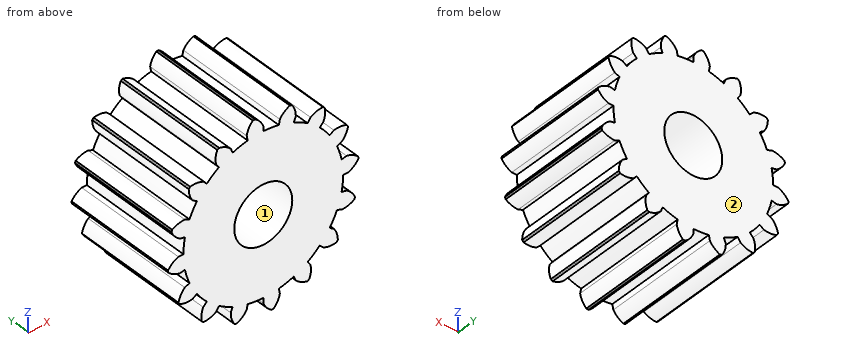
from build123d import *

# Parameters (mm, degrees)
F0_R     = 1.5875
F1_DEPTH = 6.35


with BuildPart() as f1:
    # F0 (on Front) → F1 (new body)
    with BuildSketch(Plane.XZ):
        with BuildLine():
            ThreePointArc((0, 4.653198), (-0.181622, 4.967595), (-0.451324, 5.210686))
            ThreePointArc((-0.451324, 5.210686), (-0.481995, 5.207938), (-0.512649, 5.20501))
            ThreePointArc((-0.512649, 5.20501), (-0.543285, 5.201901), (-0.573903, 5.198613))
            ThreePointArc((-0.573903, 5.198613), (-0.790998, 4.907577), (-0.907794, 4.563788))
            Line((-0.907794, 4.563788), (-0.853047, 4.288558))
            ThreePointArc((-0.853047, 4.288558), (-1.269292, 4.184294), (-1.673312, 4.039734))
            Line((-1.673312, 4.039734), (-1.780702, 4.298995))
            ThreePointArc((-1.780702, 4.298995), (-2.068813, 4.519956), (-2.411012, 4.641332))
            ThreePointArc((-2.411012, 4.641332), (-2.438297, 4.627056), (-2.465497, 4.61262))
            ThreePointArc((-2.465497, 4.61262), (-2.492612, 4.598024), (-2.51964, 4.583269))
            ThreePointArc((-2.51964, 4.583269), (-2.608835, 4.231308), (-2.585178, 3.868993))
            Line((-2.585178, 3.868993), (-2.429273, 3.635664))
            ThreePointArc((-2.429273, 3.635664), (-2.773933, 3.380047), (-3.091878, 3.091878))
            Line((-3.091878, 3.091878), (-3.290308, 3.290308))
            ThreePointArc((-3.290308, 3.290308), (-3.641046, 3.384194), (-4.003645, 3.365377))
            ThreePointArc((-4.003645, 3.365377), (-4.02339, 3.341747), (-4.042995, 3.318))
            ThreePointArc((-4.042995, 3.318), (-4.06246, 3.294139), (-4.081785, 3.270164))
            ThreePointArc((-4.081785, 3.270164), (-4.029501, 2.910861), (-3.868993, 2.585178))
            Line((-3.868993, 2.585178), (-3.635664, 2.429273))
            ThreePointArc((-3.635664, 2.429273), (-3.856268, 2.061218), (-4.039734, 1.673312))
            Line((-4.039734, 1.673312), (-4.298995, 1.780702))
            ThreePointArc((-4.298995, 1.780702), (-4.658963, 1.73322), (-4.98676, 1.577074))
            ThreePointArc((-4.98676, 1.577074), (-4.995959, 1.547687), (-5.004984, 1.518245))
            ThreePointArc((-5.004984, 1.518245), (-5.013837, 1.488752), (-5.022515, 1.459206))
            ThreePointArc((-5.022515, 1.459206), (-4.836712, 1.147262), (-4.563788, 0.907794))
            Line((-4.563788, 0.907794), (-4.288558, 0.853047))
            ThreePointArc((-4.288558, 0.853047), (-4.351521, 0.428587), (-4.372576, 0))
            Line((-4.372576, 0), (-4.653198, 0))
            ThreePointArc((-4.653198, 0), (-4.967595, -0.181622), (-5.210686, -0.451324))
            ThreePointArc((-5.210686, -0.451324), (-5.207938, -0.481995), (-5.20501, -0.512649))
            ThreePointArc((-5.20501, -0.512649), (-5.201901, -0.543285), (-5.198613, -0.573903))
            ThreePointArc((-5.198613, -0.573903), (-4.907577, -0.790998), (-4.563788, -0.907794))
            Line((-4.563788, -0.907794), (-4.288558, -0.853047))
            ThreePointArc((-4.288558, -0.853047), (-4.184294, -1.269292), (-4.039734, -1.673312))
            Line((-4.039734, -1.673312), (-4.298995, -1.780702))
            ThreePointArc((-4.298995, -1.780702), (-4.519956, -2.068813), (-4.641332, -2.411012))
            ThreePointArc((-4.641332, -2.411012), (-4.627056, -2.438297), (-4.61262, -2.465497))
            ThreePointArc((-4.61262, -2.465497), (-4.598024, -2.492612), (-4.583269, -2.51964))
            ThreePointArc((-4.583269, -2.51964), (-4.231308, -2.608835), (-3.868993, -2.585178))
            Line((-3.868993, -2.585178), (-3.635664, -2.429273))
            ThreePointArc((-3.635664, -2.429273), (-3.380047, -2.773933), (-3.091878, -3.091878))
            Line((-3.091878, -3.091878), (-3.290308, -3.290308))
            ThreePointArc((-3.290308, -3.290308), (-3.384194, -3.641046), (-3.365377, -4.003645))
            ThreePointArc((-3.365377, -4.003645), (-3.341747, -4.02339), (-3.318, -4.042995))
            ThreePointArc((-3.318, -4.042995), (-3.294139, -4.06246), (-3.270164, -4.081785))
            ThreePointArc((-3.270164, -4.081785), (-2.910861, -4.029501), (-2.585178, -3.868993))
            Line((-2.585178, -3.868993), (-2.429273, -3.635664))
            ThreePointArc((-2.429273, -3.635664), (-2.061218, -3.856268), (-1.673312, -4.039734))
            Line((-1.673312, -4.039734), (-1.780702, -4.298995))
            ThreePointArc((-1.780702, -4.298995), (-1.73322, -4.658963), (-1.577074, -4.98676))
            ThreePointArc((-1.577074, -4.98676), (-1.547687, -4.995959), (-1.518245, -5.004984))
            ThreePointArc((-1.518245, -5.004984), (-1.488752, -5.013837), (-1.459206, -5.022515))
            ThreePointArc((-1.459206, -5.022515), (-1.147262, -4.836712), (-0.907794, -4.563788))
            Line((-0.907794, -4.563788), (-0.853047, -4.288558))
            ThreePointArc((-0.853047, -4.288558), (-0.428587, -4.351521), (0, -4.372576))
            Line((0, -4.372576), (0, -4.653198))
            ThreePointArc((0, -4.653198), (0.181622, -4.967595), (0.451324, -5.210686))
            ThreePointArc((0.451324, -5.210686), (0.481995, -5.207938), (0.512649, -5.20501))
            ThreePointArc((0.512649, -5.20501), (0.543285, -5.201901), (0.573903, -5.198613))
            ThreePointArc((0.573903, -5.198613), (0.790998, -4.907577), (0.907794, -4.563788))
            Line((0.907794, -4.563788), (0.853047, -4.288558))
            ThreePointArc((0.853047, -4.288558), (1.269292, -4.184294), (1.673312, -4.039734))
            Line((1.673312, -4.039734), (1.780702, -4.298995))
            ThreePointArc((1.780702, -4.298995), (2.068813, -4.519956), (2.411012, -4.641332))
            ThreePointArc((2.411012, -4.641332), (2.438297, -4.627056), (2.465497, -4.61262))
            ThreePointArc((2.465497, -4.61262), (2.492612, -4.598024), (2.51964, -4.583269))
            ThreePointArc((2.51964, -4.583269), (2.608835, -4.231308), (2.585178, -3.868993))
            Line((2.585178, -3.868993), (2.429273, -3.635664))
            ThreePointArc((2.429273, -3.635664), (2.773933, -3.380047), (3.091878, -3.091878))
            Line((3.091878, -3.091878), (3.290308, -3.290308))
            ThreePointArc((3.290308, -3.290308), (3.641046, -3.384194), (4.003645, -3.365377))
            ThreePointArc((4.003645, -3.365377), (4.02339, -3.341747), (4.042995, -3.318))
            ThreePointArc((4.042995, -3.318), (4.06246, -3.294139), (4.081785, -3.270164))
            ThreePointArc((4.081785, -3.270164), (4.029501, -2.910861), (3.868993, -2.585178))
            Line((3.868993, -2.585178), (3.635664, -2.429273))
            ThreePointArc((3.635664, -2.429273), (3.856268, -2.061218), (4.039734, -1.673312))
            Line((4.039734, -1.673312), (4.298995, -1.780702))
            ThreePointArc((4.298995, -1.780702), (4.658963, -1.73322), (4.98676, -1.577074))
            ThreePointArc((4.98676, -1.577074), (4.995959, -1.547687), (5.004984, -1.518245))
            ThreePointArc((5.004984, -1.518245), (5.013837, -1.488752), (5.022515, -1.459206))
            ThreePointArc((5.022515, -1.459206), (4.836712, -1.147262), (4.563788, -0.907794))
            Line((4.563788, -0.907794), (4.288558, -0.853047))
            ThreePointArc((4.288558, -0.853047), (4.351521, -0.428587), (4.372576, 0))
            Line((4.372576, 0), (4.653198, 0))
            ThreePointArc((4.653198, 0), (4.967595, 0.181622), (5.210686, 0.451324))
            ThreePointArc((5.210686, 0.451324), (5.207938, 0.481995), (5.20501, 0.512649))
            ThreePointArc((5.20501, 0.512649), (5.201901, 0.543285), (5.198613, 0.573903))
            ThreePointArc((5.198613, 0.573903), (4.907577, 0.790998), (4.563788, 0.907794))
            Line((4.563788, 0.907794), (4.288558, 0.853047))
            ThreePointArc((4.288558, 0.853047), (4.184294, 1.269292), (4.039734, 1.673312))
            Line((4.039734, 1.673312), (4.298995, 1.780702))
            ThreePointArc((4.298995, 1.780702), (4.519956, 2.068813), (4.641332, 2.411012))
            ThreePointArc((4.641332, 2.411012), (4.627056, 2.438297), (4.61262, 2.465497))
            ThreePointArc((4.61262, 2.465497), (4.598024, 2.492612), (4.583269, 2.51964))
            ThreePointArc((4.583269, 2.51964), (4.231308, 2.608835), (3.868993, 2.585178))
            Line((3.868993, 2.585178), (3.635664, 2.429273))
            ThreePointArc((3.635664, 2.429273), (3.380047, 2.773933), (3.091878, 3.091878))
            Line((3.091878, 3.091878), (3.290308, 3.290308))
            ThreePointArc((3.290308, 3.290308), (3.384194, 3.641046), (3.365377, 4.003645))
            ThreePointArc((3.365377, 4.003645), (3.341747, 4.02339), (3.318, 4.042995))
            ThreePointArc((3.318, 4.042995), (3.294139, 4.06246), (3.270164, 4.081785))
            ThreePointArc((3.270164, 4.081785), (2.910861, 4.029501), (2.585178, 3.868993))
            Line((2.585178, 3.868993), (2.429273, 3.635664))
            ThreePointArc((2.429273, 3.635664), (2.061218, 3.856268), (1.673312, 4.039734))
            Line((1.673312, 4.039734), (1.780702, 4.298995))
            ThreePointArc((1.780702, 4.298995), (1.73322, 4.658963), (1.577074, 4.98676))
            ThreePointArc((1.577074, 4.98676), (1.547687, 4.995959), (1.518245, 5.004984))
            ThreePointArc((1.518245, 5.004984), (1.488752, 5.013837), (1.459206, 5.022515))
            ThreePointArc((1.459206, 5.022515), (1.147262, 4.836712), (0.907794, 4.563788))
            Line((0.907794, 4.563788), (0.853047, 4.288558))
            ThreePointArc((0.853047, 4.288558), (0.428587, 4.351521), (0, 4.372576))
            Line((0, 4.372576), (0, 4.653198))
        make_face()
        Circle(F0_R, mode=Mode.SUBTRACT)
    extrude(amount=F1_DEPTH)


solid = f1.part
Could you check a few things on this model? Use its own coordinates, in mm. Face numbers are marked on the shaded views. Give positions to 0.01 mm unless a question says otherwise; leave off trailing zeros. Loops run counter-clockwise (first coordinate to the right, second up) from the corner with the lowest first, then second, coordinate; pieces in that order, holes last. Notation, with made-up numbers: (-1, -7.5) -> (56, -7.5) arc R7 cw to (56, 5.5) -> close; hole circle Ø3 at (82.5, -16.75). An arc over 180 degrees is marked (long way). Return JSON: item names as keys, results as strings.
Item 1: I need wall thicknesses on L1, parallel to Z at x = -4.5, y = -5.25; L2, parallel to X at y = -4.5, z = 4.75; L3, parallel to X at y = -1, z = -1.25. Which ranges of each line are inside material? Lowest first, please. Write a range as from..to.
Geometry results:
{"L1": "z = -2.55..-2.03, -0.9..0, 0.9..1.77", "L2": "x = -0.86..-0.04, 1.05..1.7", "L3": "x = -4.19..-0.98, 0.98..4.91"}
Item 2: If we section it at C-C on z = 2.75: List the corners of the cut face in (x, y) for me.
Geometry results:
{"outline": "(-3.97, -6.35) -> (3.4, -6.35) -> (3.4, 0) -> (-3.97, 0) -> close"}
Item 3: I'm going to push flat-ended pins straight in: pin 1 (1 mm diameter, centred on y = -4.5, z = -2, fed in from -X); pin 2 (3 mm diameter, centred on y = -3, z = 3.5, fed in from -X). Where does each tip first touch, or does it pass through?
Geometry results:
{"pin 1": "stops at x = -4.64", "pin 2": "stops at x = -4.08"}
Item 4: We'd pull the mould along X, two halves only. Please class the marked faces 1 and 2: +X half, -X half, draft (parallel to the pull), parting line (faces both ways), or undercut.
Geometry results:
{"face 1": "undercut", "face 2": "draft"}
Item 5: If we section it at B-B on z = -2: List the corners of the cut face in (x, y) for me.
Geometry results:
{"outline": "(-4.48, -6.35) -> (3.89, -6.35) -> (3.89, 0) -> (-4.48, 0) -> close"}
Item 6: If we section it at A-A on x = -0.25: List the corners of the cut face in (y, z) for me.
Geometry results:
{"outline": "(-6.35, -4.37) -> (0, -4.37) -> (0, -1.57) -> (-6.35, -1.57) -> close; (-6.35, 1.57) -> (0, 1.57) -> (0, 5.04) -> (-6.35, 5.04) -> close"}
